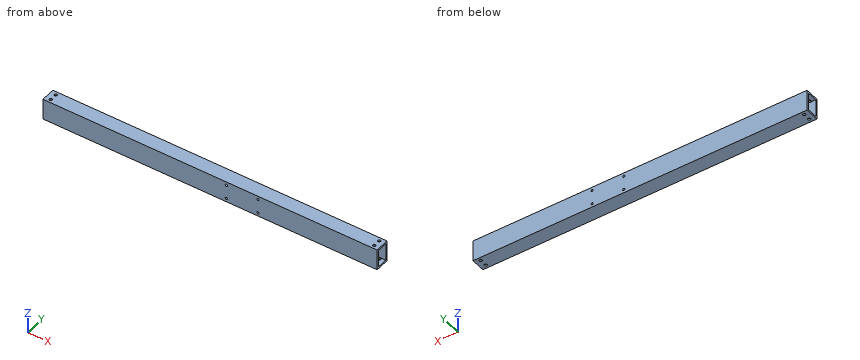
from build123d import *

# Parameters (mm, degrees)
SKETCH1_W           = 38.1
SKETCH1_H           = 25.4
SKETCH1_W_2         = 31.75
SKETCH1_H_2         = 19.05
BOSS_EXTRUDE1_DEPTH = 301.625
SKETCH2_R           = 2.4892
CUT_EXTRUDE1_DEPTH  = 39.1
SKETCH4_R           = 2.0193
CUT_EXTRUDE2_DEPTH  = 26.4


with BuildPart() as part:
    # Sketch1 → Boss-Extrude1 (new body, symmetric)
    with BuildSketch(Plane(origin=(0, 0, 0), x_dir=(0, 0, -1), z_dir=(1, 0, 0))):
        Rectangle(SKETCH1_W, SKETCH1_H)
        Rectangle(SKETCH1_W_2, SKETCH1_H_2, mode=Mode.SUBTRACT)
    extrude(amount=BOSS_EXTRUDE1_DEPTH, both=True)

    # Sketch2 → Cut-Extrude1 (cut, through all)
    with BuildSketch(Plane.XY.offset(19.05)):
        with Locations((-292.1, 6.35)):
            Circle(SKETCH2_R)
        with Locations((-292.1, -6.35)):
            Circle(SKETCH2_R)
    cut_extrude1 = extrude(amount=-CUT_EXTRUDE1_DEPTH, mode=Mode.SUBTRACT)

    # Mirror1: Cut-Extrude1 across plane
    add(cut_extrude1.mirror(Plane(origin=(0, 0, 0), x_dir=(0, 0, 1), z_dir=(1, 0, 0))), mode=Mode.SUBTRACT)

    # Sketch4 → Cut-Extrude2 (cut, through all)
    with BuildSketch(Plane.XZ.offset(12.7)):
        with Locations((86.5502, -12.7)):
            Circle(SKETCH4_R)
        with Locations((86.5502, 12.7)):
            Circle(SKETCH4_R)
        with Locations((29.4002, 12.7)):
            Circle(SKETCH4_R)
        with Locations((29.4002, -12.7)):
            Circle(SKETCH4_R)
    extrude(amount=-CUT_EXTRUDE2_DEPTH, mode=Mode.SUBTRACT)


solid = part.part
Check sheet for the modelled part. Datum: model origin and axes. Units: mm. Round coordinates to 2 decimals unless told otherwise and drop trailing zeros. Loops run counter-clockwise (first coordinate to the right, second up) from the corner with the lowest first, then second, coordinate; pieces in that order, holes last. Notation, with made-up numbers: (88, -12) - (132, -12) arc R25 ccw to (132, 17) - close; hole circle Ø3 at (3, 0). An arc over 180 degrees is marked (long way). Answer as CSV lines item,"result". Start each with the question number.
Item 1: Depth check by flat-ended pin: P1, Ø4.5, axis at x = 29.4, z = 12.7, coming from the -Y side. Enter the tip coordinate at first touch or a pass-through.
Item 2: Scan lines: line 1 (Y direction, x = 292.1, z = -18.1); line 2 (Z direction, x = -143, y = -4) (3 decimals); line 3 (Y direction, x = 54.5, z = 3) (3 decimals). Record each from-to range of solid material in increasing order. Write a range as [from, to].
Item 3: Section check B-B (z = 3). Record the boundary of the cut face in (x, y) (3 decimals), and give its area (3 significant figures).
Item 4: Section check A-A (x = -54.5). Record the boundary of the cut face in (y, z) (3 decimals), and give its area (3 significant figures).
Report:
1,P1,"stops at y = -12.7"
2,line 1,"y = [-12.7, -8.84], [-3.86, 3.86], [8.84, 12.7]"
2,line 2,"z = [-19.05, -15.875], [15.875, 19.05]"
2,line 3,"y = [-12.7, -9.525], [9.525, 12.7]"
3,outline,"(-301.625, -12.7) - (301.625, -12.7) - (301.625, -9.525) - (-301.625, -9.525) - close; (-301.625, 9.525) - (301.625, 9.525) - (301.625, 12.7) - (-301.625, 12.7) - close"
3,area,"3,830 mm2"
4,outline,"(-12.7, -19.05) - (12.7, -19.05) - (12.7, 19.05) - (-12.7, 19.05) - close; hole (-9.525, -15.875) - (9.525, -15.875) - (9.525, 15.875) - (-9.525, 15.875) - close"
4,area,"363 mm2"
